Autodesk Inventor part; units mm, degrees
ref_plane "YZ Plane" through (0, 0, 0) normal (1, 0, 0) x (0, 1, 0)
ref_plane "XZ Plane" through (0, 0, 0) normal (0, 1, 0) x (-1, 0, 0)
ref_plane "XY Plane" through (0, 0, 0) normal (0, 0, 1) x (1, 0, 0)
sketch "Sketch1" plane through (0, 0, 0) normal (0, 0, 1) x (1, 0, 0)
  circle A0 centre (0, 0) radius 13.25
  dimension "d0" = 26.5
extrude "Extrusion1" add sketch "Sketch1" along normal blind 4
sketch "Sketch2" plane through (0, 0, 4) normal (0, 0, 1) x (1, 0, 0)
  circle A0 centre (0, 0) radius 15
  dimension "d3" = 30
extrude "Extrusion2" add sketch "Sketch2" along normal blind 2
chamfer "Chamfer1" distance 1 angle 45 1 edges at (-15, 0, 6)
chamfer "Chamfer2" distance 1 angle 45 1 edges at (-13.25, 0, 0)
properties part number "Plug21mm_3DPrint"
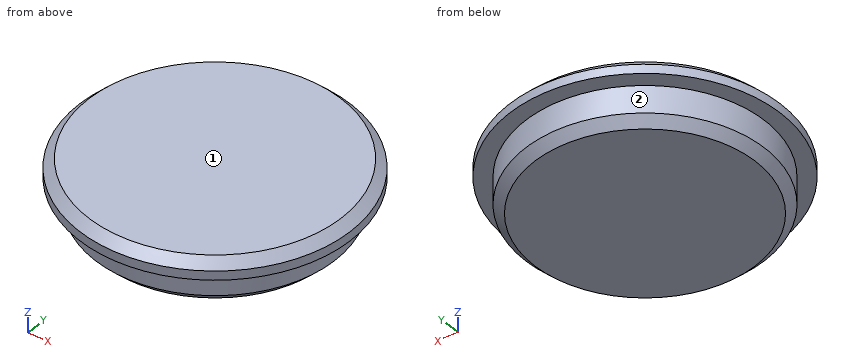
The listing builds one solid part. Answer for the finished solid, in the listing's coordinates (mm). Face numbers are marked on the shaded views. A direction names the side the tool comes from. Give positions to 0.01 mm unless a question says otherwise; leave off trailing zeros. Order: outer loops, then holes, each group sorted by start corner. A loop starts at its lowest first (then second) coordinate and runs counter-clockwise, first axis right, second up. Notation, with made-up numbers: (15, 2.5) - (53, 2.5) arc R22 ccw to (53, 25.5) - close; hole circle Ø11 at (31.5, 73.25). An arc over 180 degrees is marked (long way). Answer in a Markdown table with one row per item. Add a question column.
Q1. Which of the six approach directions +Z, -Z, +X, -X, +Y, -Y give full straight-line access (tool end or side, diameter ignored) to the marked faces 1 and 2?
Q2. The part is cut by section D-D (z = 3.65). Determine the outline of the cut face in (x, y).
Q3. The part is cut by section A-A (y = 0). Determine the outline of the cut face in (x, z).
Q4. Find the intervals of material crossed by line 1 along Z through (x, y) = (2.25, 13.5); line 2 along Y through (x, z) = (0.25, 4.6); line 3 along Y through (x, z) = (6, 5.1), in increasing order. Write a range as [from, to].
Q5. The part is cut by section C-C (z = 5.55). Determine the outline of the cut face in (x, y), then the cut area to 3 significant figures.
Q6. Given P1, Ø3, axis at x = 5.5, z = 4.5, coming from the -Y side; P2, Ø3, axis at y = -10, z = 2, coming from the -X side; P3, Ø1.5, axis at y = -2.5, z = 1, coming from the +X side, each flat-ended and moving along its own axis, determine where each tip first touches the part or whether it passes through.
Determined:
| question | item | result |
|---|---|---|
| 1 | face 1 | +Z, +X, -X, +Y, -Y |
| 1 | face 2 | -Z |
| 2 | outline | circle Ø26.5 at (0, 0) |
| 3 | outline | (-15, 4) - (-13.25, 4) - (-13.25, 1) - (-12.25, 0) - (12.25, 0) - (13.25, 1) - (13.25, 4) - (15, 4) - (15, 5) - (14, 6) - (-14, 6) - (-15, 5) - close |
| 4 | line 1 | z = [4, 6] |
| 4 | line 2 | y = [-15, 15] |
| 4 | line 3 | y = [-13.64, 13.64] |
| 5 | outline | circle Ø28.9 at (0, 0) |
| 5 | area | 656 mm² |
| 6 | P1 | stops at y = -14.46 |
| 6 | P2 | stops at x = -10.16 |
| 6 | P3 | stops at x = 13.13 |
